Check sheet for the drawn part. Datum: minimum x, y, z corner. Units: mm. Round coordinates to 2 decimals unless told otherwise and drop trailing zeros. Write each loop counter-clockwise with the first axis right and the second up, starting at its lowest first coordinate (ties: lowest second). Pieces come first, ordered by that corner, then holes. Notation, with made-up numbers: M 41.5,85.25 L 57.5,85.25 A4 cw 57.5,89.25 Z; hole C 25.5,-15 d10. An arc over 180 degrees is marked long. One line per item, written item: value. Start each with the question number.
1. Depth check by flat-ended pin: P1, Ø2, axis at y = 11, z = 2, coming from the -X side. Enter the tip coordinate at first touch or a pass-through.
2. Section check B-B (y = 12.75). Record the boundary of the cut face in (x, z).
3. Section check C-C (y = 2.5). Record the boundary of the cut face in (x, z) (1 decimal).
4. Section check D-D (x = 22). Record the boundary of the cut face in (y, z), and give its area (3 significant figures).
5. Scan lines: probe 1 along X at (y, z) = (8.75, 2.05); probe 2 along X at (y, z) = (9.25, 2.35); probe 3 along Y at (x, z) = (78.5, 0.65). Record each from-to range of solid material in increasing order. Write a range as [from, to].
6. Section check A-A (z = 2.05). Record the boundary of the cut face in (x, y) (1 decimal), and give its area (3 significant figures).
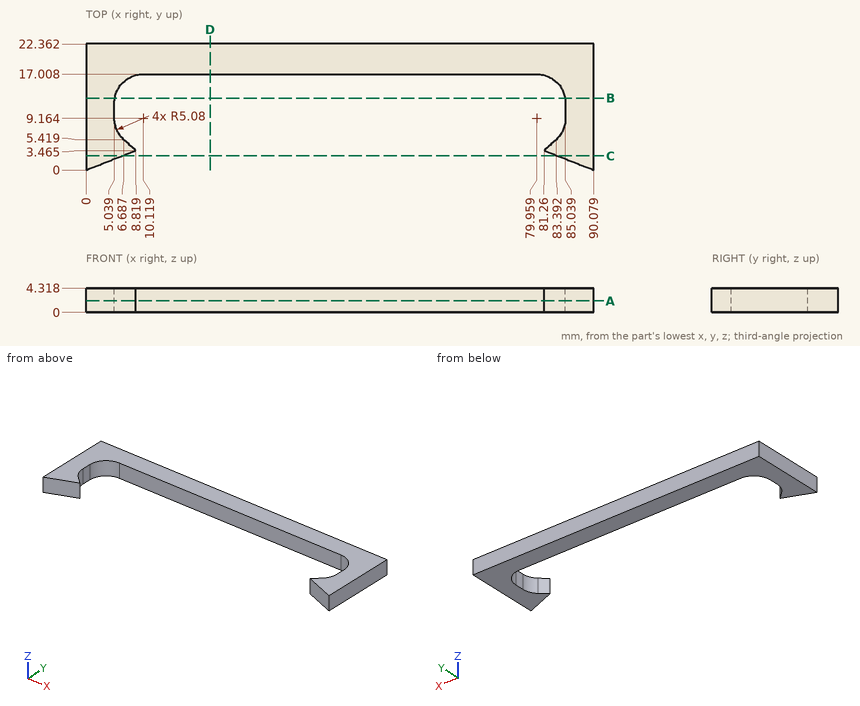
Result sheet:
1. P1: stops at x = 0
2. outline: M 0,0 L 5.11,0 L 5.11,4.32 L 0,4.32 Z; M 84.97,0 L 90.08,0 L 90.08,4.32 L 84.97,4.32 Z
3. outline: M 0,0 L 6.4,0 L 6.4,4.3 L 0,4.3 Z; M 83.7,0 L 90.1,0 L 90.1,4.3 L 83.7,4.3 Z
4. outline: M 17.01,0 L 22.36,0 L 22.36,4.32 L 17.01,4.32 Z
4. area: 23.1 mm2
5. probe 1: x = [0, 5.06], [85.02, 90.08]
5. probe 2: x = [0, 5.04], [85.04, 90.08]
5. probe 3: y = [17.01, 22.36]
6. outline: M 0,0 L 8.8,3.5 L 6.7,5.4 A5.1 cw 5,9.2 L 5,11.9 A5.1 cw 10.1,17 L 80,17 A5.1 cw 85,11.9 L 85,9.2 A5.1 cw 83.4,5.4 L 81.3,3.5 L 90.1,0 L 90.1,22.4 L 0,22.4 Z
6. area: 675 mm2
